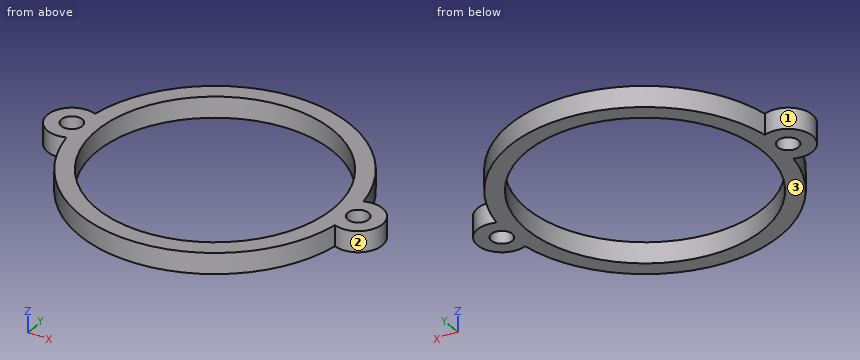
from build123d import *

# Parameters (mm, degrees)
SKETCH_R   = 17
SKETCH_R_2 = 1.5
PAD_DEPTH  = 3


with BuildPart() as part:
    # Sketch → Pad (new body)
    with BuildSketch(Plane.XY):
        with BuildLine():
            ThreePointArc((19.22561, 3.259744), (0, 19.5), (-19.22561, 3.259744))
            ThreePointArc((-19.22561, 3.259744), (-24, 0), (-19.22561, -3.259744))
            ThreePointArc((-19.22561, -3.259744), (0, -19.5), (19.22561, -3.259744))
            ThreePointArc((19.22561, -3.259744), (24, 0), (19.22561, 3.259744))
        make_face()
        Circle(SKETCH_R, mode=Mode.SUBTRACT)
        with Locations((20.5, 0)):
            Circle(SKETCH_R_2, mode=Mode.SUBTRACT)
        with Locations((-20.5, 0)):
            Circle(SKETCH_R_2, mode=Mode.SUBTRACT)
    extrude(amount=PAD_DEPTH)


solid = part.part
Design review of the part built by this model. Coordinates are the model's own, in mm. Face numbers are marked on the shaded views. Give positions to 0.01 mm unless a question says otherwise; leave off trailing zeros. Loops run counter-clockwise (first coordinate to the right, second up) from the corner with the lowest first, then second, coordinate; pieces in that order, holes last. Notation, with made-up numbers: M -15,-17 L -10,-17 A30 ccw -10,19 Z; hole C 4,-12.75 d8. An arc over 180 degrees is marked long. One line per question, with ' | ' between items. Start each with the question number.
1. Insertion check: P1, Ø1.5, axis at x = 4, z = 2, coming from the -Y side; P2, Ø1, axis at y = -12, z = 1.5, coming from the -X side; P3, Ø4, axis at x = -15, y = -9.5, coming from the -Z side; P4, Ø1.8, axis at x = -20.5, y = 0, coming from the +Z side. Each pin has a flat end and moves straight along its axis. Give the tip position at first contact, or say it passes through.
2. Add section C-C (z = 1.3). Write out the cut boundary in (x, y), plus the area to 3 significant figures.
3. Add section D-D (y = -8.5). Write out the cut boundary in (x, z).
4. Add section A-A (x = 0). Write out the cut boundary in (y, z), plus the area to 3 significant figures.
5. Add section B-B (y = 0). Write out the cut boundary in (x, z), plus the area to 3 significant figures.
6. To check wall thickness, follow L1, parallel to Y at x = 20.5, z = 0.8; L2, parallel to X at y = -4.5, z = 0.6; L3, parallel to Y at x = 1, z = 0.1. State the ranges of each line that lie inside material, in increasing order.
7. The part is to be moulded in two halves that separate along X. For the marked faces 1, 2 and 3, say which applies: released by +X, released by -X, zero draft, split by the parting line, or undercut.
Worked out:
1) P1: stops at y = -19.23 | P2: stops at x = -15.75 | P3: stops at z = 0 | P4: passes through
2) outline: M -19.23,-3.26 A19.5 ccw 19.23,-3.26 A3.5 ccw long 19.23,3.26 A19.5 ccw -19.23,3.26 A3.5 ccw long Z; hole C -20.5,0 d3; hole C 0,0 d34; hole C 20.5,0 d3 | area: 326 mm²
3) outline: M -17.55,0 L -14.72,0 L -14.72,3 L -17.55,3 Z; M 14.72,0 L 17.55,0 L 17.55,3 L 14.72,3 Z
4) outline: M -19.5,0 L -17,0 L -17,3 L -19.5,3 Z; M 17,0 L 19.5,0 L 19.5,3 L 17,3 Z | area: 15.0 mm²
5) outline: M -24,0 L -22,0 L -22,3 L -24,3 Z; M -19,0 L -17,0 L -17,3 L -19,3 Z; M 17,0 L 19,0 L 19,3 L 17,3 Z; M 22,0 L 24,0 L 24,3 L 22,3 Z | area: 24.0 mm²
6) L1: y = -3.5 to -1.5, 1.5 to 3.5 | L2: x = -18.97 to -16.39, 16.39 to 18.97 | L3: y = -19.47 to -16.97, 16.97 to 19.47
7) face 1: undercut | face 2: undercut | face 3: zero draft
